Answer from the drawing. Dimensions are ordinates in mm from the lowest x, y and z of the part. Coordinates: 2 decimals unless noted, no trailing zeros. Loops run counter-clockwise (first coordinate to the right, second up) from the corner with the lowest first, then second, coordinate; pieces in that order, holes last. Notation, with made-up numbers: (54, -4.5) -> (103, -4.5) arc R26 ccw to (103, 19.5) -> close; hole circle Ø10 at (11, -8). An arc over 180 degrees is marked (long way). Use a Markdown table: item, result.
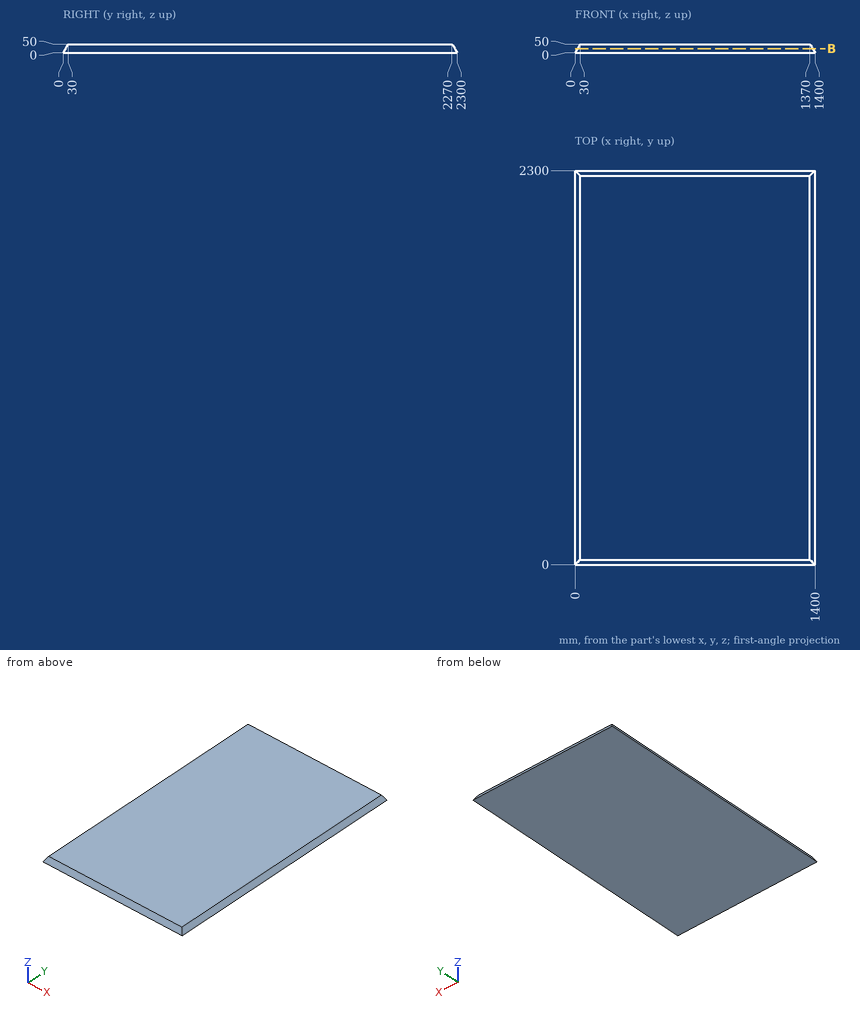
Q1. Given pin 1 Ø10 at (x, z) = (1096.5, 15.5) entering from -Y; pin 2 Ø3 at (y, z) = (1696, 16) entering from -X; pin 3 Ø10 at (x, z) = (761, 38) entering from +Y, each flat-ended and moving along its own axis, determine where each tip first touches the part or whether it passes through.
Solved:
| item | result |
|---|---|
| pin 1 | y = 6.3 |
| pin 2 | x = 8.7 |
| pin 3 | y = 2280.2 |
Q2. Section B-B on z = 23 is taken. Determine the outline of the cut face in (x, y).
Solved:
| item | result |
|---|---|
| outline | (13.8, 13.8) -> (1386.2, 13.8) -> (1386.2, 2286.2) -> (13.8, 2286.2) -> close |
Q3. Consider line 1 (Y direction, x = 1322.5, z = 6); line 2 (Y direction, x = 655, z = 8.5); line 3 (X direction, y = 415.5, z = 4). Determine where each line is inside the solid, lowest interval first. Write a range as [from, to].
Solved:
| item | result |
|---|---|
| line 1 | [3.6, 2296.4] |
| line 2 | [5.1, 2294.9] |
| line 3 | [2.4, 1397.6] |
